Verification items for the finished model (mm, model axes). Face numbers are marked on the shaded views. A direction names the side the tool comes from. Round coordinates to 2 decimals unless told otherwise and drop trailing zeros. Order: outer loops, then holes, each group sorted by start corner. A loop starts at its lowest first (then second) coordinate and runs counter-clockwise, first axis right, second up. Notation, with made-up numbers: M 35,79 L 47,79 A9 cw 47,88 Z; hole C 25,51.25 d1. An arc over 180 degrees is marked long. Answer as a JSON object with one key per item and string values. Group by question number.
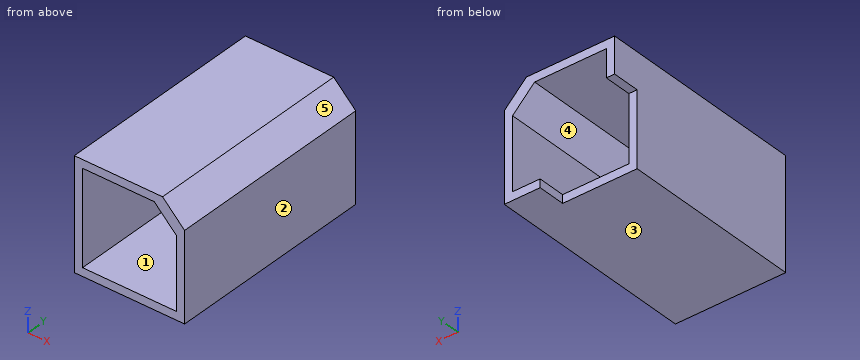
```python
from build123d import *

# Parameters (mm, degrees)
F0_W     = 20
F0_H     = 20
F0_W_2   = 17
F0_H_2   = 17
F1_DEPTH = 38
F2_SIZE  = 4
F4_DEPTH = 5


with BuildPart() as f1:
    # F0 (on Front) → F1 (new body)
    with BuildSketch(Plane.XZ):
        with Locations((10, 10)):
            Rectangle(F0_W, F0_H)
        with Locations((10, 10)):
            Rectangle(F0_W_2, F0_H_2, mode=Mode.SUBTRACT)
    extrude(amount=F1_DEPTH)

    # F2
    f2_edges = [f1.edges().sort_by_distance(p)[0] for p in [
        (20, -19, 20),
        (18.5, -19, 18.5),
    ]]
    chamfer(f2_edges, length=F2_SIZE)

    # F1_face (on face) + F3 (on Front) → F4 (cut)
    with BuildSketch(Plane(origin=(9.891892, -38, 9.891892), x_dir=(1, 0, 0), z_dir=(0, -1, 0))):
        Polygon((10.108108, -9.891892), (10.108108, 6.108108), (6.108108, 10.108108), (-9.891892, 10.108108), (-9.891892, -9.891892), align=None)
        Polygon((-8.391892, 8.608108), (4.608108, 8.608108), (8.608108, 4.608108), (8.608108, -8.391892), (-8.391892, -8.391892), align=None, mode=Mode.SUBTRACT)
    with BuildSketch(Plane.XZ):
        Polygon((0, 13.5), (0, 0), (13.5, 0), (13.5, 1.5), (1.5, 1.5), (1.5, 13.5), align=None)
    extrude(amount=F4_DEPTH, mode=Mode.SUBTRACT)


solid = f1.part
```
Q1. Cross-section at D-D, the plane y = -3.5. Record the cut outline in (x, z).
Q2. Thickness scan on line 1 (Z direction, x = 13.5, y = -33); line 2 (Y direction, x = 1, z = 5.25). Record the ranges inside material, lowest first. Write a range as from..to.
Q3. Cross-section at B-B, the plane x = 17.75. Record the cut outline in (y, z), then the cut area to 3 significant figures.
Q4. Cross-section at C-C, the plane y = -33.5. Record the cut outline in (x, z).
Q5. Gauge pin test, flat ends, axial feed: pin 1 Ø1.6 at (y, z) = (-3.5, 1) entering from -X; pin 2 Ø0.8 at (x, y) = (0.5, -3) entering from -Z. Record the tip position at first contact, or that the pin passes through.
Q6. Tool access check on the marked faces 1 and 2. Record the directions out of +Z, -Z, +X, -X, +Y, -Y that give a thin tool (end or side, any length) a straight path to the whole face; none if there is none.
Q7. Release check for a two-part mould opening along Z. For the marked faces 3, 4 and 5 record: released by +Z, released by -Z, zero draft, split by the parting line, or undercut.
Q8. Cross-section at A-A, the plane z = 14. Record the cut outline in (x, y).
Conclusion:
{
 "1": {"outline": "M 0,13.5 L 1.5,13.5 L 1.5,18.5 L 14.5,18.5 L 18.5,14.5 L 18.5,1.5 L 13.5,1.5 L 13.5,0 L 20,0 L 20,16 L 16,20 L 0,20 Z"},
 "2": {"line 1": "0..1.5, 18.5..20", "line 2": "-38..-5"},
 "3": {"outline": "M -38,0 L 0,0 L 0,1.5 L -38,1.5 Z; M -38,15.25 L 0,15.25 L 0,18.25 L -38,18.25 Z", "area": "171 mm2"},
 "4": {"outline": "M 0,0 L 20,0 L 20,16 L 16,20 L 0,20 Z; hole M 1.5,1.5 L 18.5,1.5 L 18.5,14.5 L 14.5,18.5 L 1.5,18.5 Z"},
 "5": {"pin 1": "x = 13.5", "pin 2": "z = 13.5"},
 "6": {"face 1": "+Y, -Y", "face 2": "+Z, -Z, +X, +Y, -Y"},
 "7": {"face 3": "released by -Z", "face 4": "undercut", "face 5": "released by +Z"},
 "8": {"outline": "M 0,-38 L 1.5,-38 L 1.5,0 L 0,0 Z; M 18.5,-38 L 20,-38 L 20,0 L 18.5,0 Z"}
}
